Read the model definition and answer for the solid it produces. Units are mm, in the model's axes. Face numbers are marked on the shaded views. A direction names the side the tool comes from. Give positions to 0.01 mm unless a question says otherwise; leave off trailing zeros. Write each loop counter-clockwise with the first axis right and the second up, starting at its lowest first coordinate (ties: lowest second). Pieces come first, ordered by that corner, then holes. Notation, with made-up numbers: (19, 15) - (54, 15) arc R19 ccw to (54, 31) - close; hole circle Ø8 at (29.5, -4). An arc over 180 degrees is marked (long way). Answer as CSV lines item,"result".
```python
from build123d import *

# Parameters (mm, degrees)
SKETCH1_W            = 6
SKETCH1_H            = 6
BOSS_EXTRUDE1_DEPTH  = 3.61
SKETCH2_W            = 0.7
SKETCH2_H            = 0.3
BOSS_EXTRUDE2_DEPTH  = 2
SKETCH3_W            = 0.7
SKETCH3_H            = 1.35
BOSS_EXTRUDE3_DEPTH  = 1.15
SKETCH4_W            = 0.7
SKETCH4_H            = 0.3
BOSS_EXTRUDE4_DEPTH  = 2
SKETCH5_W            = 0.7
SKETCH5_H            = 1.35
BOSS_EXTRUDE5_DEPTH  = 1.15
SKETCH6_W            = 0.7
SKETCH6_H            = 0.3
BOSS_EXTRUDE6_DEPTH  = 2
SKETCH7_W            = 0.7
SKETCH7_H            = 1.35
BOSS_EXTRUDE7_DEPTH  = 1.15
SKETCH8_W            = 0.7
SKETCH8_H            = 0.3
BOSS_EXTRUDE8_DEPTH  = 2
SKETCH9_W            = 0.7
SKETCH9_H            = 1.35
BOSS_EXTRUDE9_DEPTH  = 1.15
CUT_EXTRUDE1_REACH   = 10.374
SKETCH10_W           = 1.15
SKETCH10_H           = 1.05
SKETCH11_W           = 1.15
SKETCH11_H           = 1.05
CUT_EXTRUDE2_DEPTH   = 8.923010791
CUT_EXTRUDE3_REACH   = 10.374
SKETCH12_W           = 1.15
SKETCH12_H           = 1.05
SKETCH13_W           = 1.15
SKETCH13_H           = 1.05
CUT_EXTRUDE4_DEPTH   = 8.923010791
SKETCH14_W           = 0.5
SKETCH14_H           = 0.4
SKETCH15_W           = 0.5
SKETCH15_H           = 0.4
SKETCH16_W           = 0.5
SKETCH16_H           = 0.4
SKETCH17_W           = 0.5
SKETCH17_H           = 0.4
FILLET1_R            = 0.25
FILLET2_R            = 0.55
SKETCH19_R           = 1.75
BOSS_EXTRUDE10_DEPTH = 1.4
FILLET4_R            = 0.1


with BuildPart() as part:
    # Sketch1 → Boss-Extrude1 (new body)
    with BuildSketch(Plane.XY):
        Rectangle(SKETCH1_W, SKETCH1_H)
    extrude(amount=-BOSS_EXTRUDE1_DEPTH)

    # Sketch2 → Boss-Extrude2 (add)
    with BuildSketch(Plane.XZ.offset(3)):
        with Locations((-2.25, -2.41)):
            Rectangle(SKETCH2_W, SKETCH2_H)
    extrude(amount=BOSS_EXTRUDE2_DEPTH)

    # Sketch3 → Boss-Extrude3 (add)
    with BuildSketch(Plane(origin=(0, 0, -2.56), x_dir=(-1, 0, 0), z_dir=(0, 0, -1))):
        with Locations((2.25, -4.325)):
            Rectangle(SKETCH3_W, SKETCH3_H)
    extrude(amount=BOSS_EXTRUDE3_DEPTH)

    # Sketch4 → Boss-Extrude4 (add)
    with BuildSketch(Plane.XZ.offset(3)):
        with Locations((2.25, -2.41)):
            Rectangle(SKETCH4_W, SKETCH4_H)
    extrude(amount=BOSS_EXTRUDE4_DEPTH)

    # Sketch5 → Boss-Extrude5 (add)
    with BuildSketch(Plane(origin=(0, 0, -2.56), x_dir=(-1, 0, 0), z_dir=(0, 0, -1))):
        with Locations((-2.25, -4.325)):
            Rectangle(SKETCH5_W, SKETCH5_H)
    extrude(amount=BOSS_EXTRUDE5_DEPTH)

    # Sketch6 → Boss-Extrude6 (add)
    with BuildSketch(Plane(origin=(0, 3, 0), x_dir=(-1, 0, 0), z_dir=(0, 1, 0))):
        with Locations((2.25, -2.41)):
            Rectangle(SKETCH6_W, SKETCH6_H)
    extrude(amount=BOSS_EXTRUDE6_DEPTH)

    # Sketch7 → Boss-Extrude7 (add)
    with BuildSketch(Plane(origin=(0, 0, -2.56), x_dir=(-1, 0, 0), z_dir=(0, 0, -1))):
        with Locations((2.25, 4.325)):
            Rectangle(SKETCH7_W, SKETCH7_H)
    extrude(amount=BOSS_EXTRUDE7_DEPTH)

    # Sketch8 → Boss-Extrude8 (add)
    with BuildSketch(Plane(origin=(0, 3, 0), x_dir=(-1, 0, 0), z_dir=(0, 1, 0))):
        with Locations((-2.25, -2.41)):
            Rectangle(SKETCH8_W, SKETCH8_H)
    extrude(amount=BOSS_EXTRUDE8_DEPTH)

    # Sketch9 → Boss-Extrude9 (add)
    with BuildSketch(Plane(origin=(0, 0, -2.56), x_dir=(-1, 0, 0), z_dir=(0, 0, -1))):
        with Locations((-2.25, 4.325)):
            Rectangle(SKETCH9_W, SKETCH9_H)
    extrude(amount=BOSS_EXTRUDE9_DEPTH)

    # Sketch10 → Cut-Extrude1 (cut, up to next)
    with BuildSketch(Plane.ZY.offset(2.6), mode=Mode.PRIVATE) as cut_extrude1_sk1:
        with Locations((-2.835, -4.475)):
            Rectangle(SKETCH10_W, SKETCH10_H)
    cut_extrude1_tool1 = extrude(cut_extrude1_sk1.sketch, amount=-CUT_EXTRUDE1_REACH, mode=Mode.PRIVATE) & part.part
    add(cut_extrude1_tool1.solids().sort_by_distance((-2.6, -4.475, -2.835))[0], mode=Mode.SUBTRACT)

    # Sketch11 → Cut-Extrude2 (cut, through all)
    with BuildSketch(Plane.ZY.offset(-1.9)):
        with Locations((-2.835, -4.475)):
            Rectangle(SKETCH11_W, SKETCH11_H)
    extrude(amount=-CUT_EXTRUDE2_DEPTH, mode=Mode.SUBTRACT)

    # Sketch12 → Cut-Extrude3 (cut, up to next)
    with BuildSketch(Plane.ZY.offset(2.6), mode=Mode.PRIVATE) as cut_extrude3_sk1:
        with Locations((-2.835, 4.475)):
            Rectangle(SKETCH12_W, SKETCH12_H)
    cut_extrude3_tool1 = extrude(cut_extrude3_sk1.sketch, amount=-CUT_EXTRUDE3_REACH, mode=Mode.PRIVATE) & part.part
    add(cut_extrude3_tool1.solids().sort_by_distance((-2.6, 4.475, -2.835))[0], mode=Mode.SUBTRACT)

    # Sketch13 → Cut-Extrude4 (cut, through all)
    with BuildSketch(Plane.ZY.offset(-1.9)):
        with Locations((-2.835, 4.475)):
            Rectangle(SKETCH13_W, SKETCH13_H)
    extrude(amount=-CUT_EXTRUDE4_DEPTH, mode=Mode.SUBTRACT)

    # Sketch14 → Revolve1 (revolve)
    with BuildSketch(Plane(origin=(0, -2.165, 0), x_dir=(-1, 0, 0), z_dir=(0, 1, 0))):
        with Locations((-2.415, 0.2)):
            Rectangle(SKETCH14_W, SKETCH14_H)
    revolve(axis=Axis((2.165, -2.165, 0), (0, 0, 1)))

    # Sketch15 → Revolve2 (revolve)
    with BuildSketch(Plane(origin=(0, -2.165, 0), x_dir=(-1, 0, 0), z_dir=(0, 1, 0))):
        with Locations((1.915, 0.2)):
            Rectangle(SKETCH15_W, SKETCH15_H)
    revolve(axis=Axis((-2.165, -2.165, 0), (0, 0, 1)))

    # Sketch16 → Revolve3 (revolve)
    with BuildSketch(Plane(origin=(0, 2.165, 0), x_dir=(-1, 0, 0), z_dir=(0, 1, 0))):
        with Locations((1.915, 0.2)):
            Rectangle(SKETCH16_W, SKETCH16_H)
    revolve(axis=Axis((-2.165, 2.165, 0), (0, 0, 1)))

    # Sketch17 → Revolve4 (revolve)
    with BuildSketch(Plane(origin=(0, 2.165, 0), x_dir=(-1, 0, 0), z_dir=(0, 1, 0))):
        with Locations((-2.415, 0.2)):
            Rectangle(SKETCH17_W, SKETCH17_H)
    revolve(axis=Axis((2.165, 2.165, 0), (0, 0, 1)))

    # Fillet1
    fillet1_edges = [part.edges().sort_by_distance(p)[0] for p in [
        (2.25, 3.65, -2.56),
        (-2.25, -3.95, -3.41),
        (2.25, -3.95, -3.41),
        (-2.25, 3.95, -3.41),
        (2.25, 3.95, -3.41),
        (-2.25, -3.65, -2.56),
        (2.25, -3.65, -2.56),
        (-3, -3, -1.805),
        (-3, 3, -1.805),
        (3, 3, -1.805),
        (3, -3, -1.805),
        (-2.25, 3.65, -2.56),
    ]]
    fillet(fillet1_edges, radius=FILLET1_R)

    # Fillet2
    fillet2_edges = [part.edges().sort_by_distance(p)[0] for p in [
        (2.25, 3.65, -3.71),
        (-2.25, -3.95, -2.26),
        (2.25, -3.95, -2.26),
        (-2.25, 3.95, -2.26),
        (2.25, 3.95, -2.26),
        (-2.25, -3.65, -3.71),
        (2.25, -3.65, -3.71),
        (-2.25, 3.65, -3.71),
    ]]
    fillet(fillet2_edges, radius=FILLET2_R)

    # Sketch19 → Boss-Extrude10 (add)
    with BuildSketch(Plane.XY):
        Circle(SKETCH19_R)
    extrude(amount=BOSS_EXTRUDE10_DEPTH)

    # Fillet4
    fillet4_edges = [part.edges().sort_by_distance(p)[0] for p in [
        (-1.75, 0, 1.4),
    ]]
    fillet(fillet4_edges, radius=FILLET4_R)


solid = part.part
```
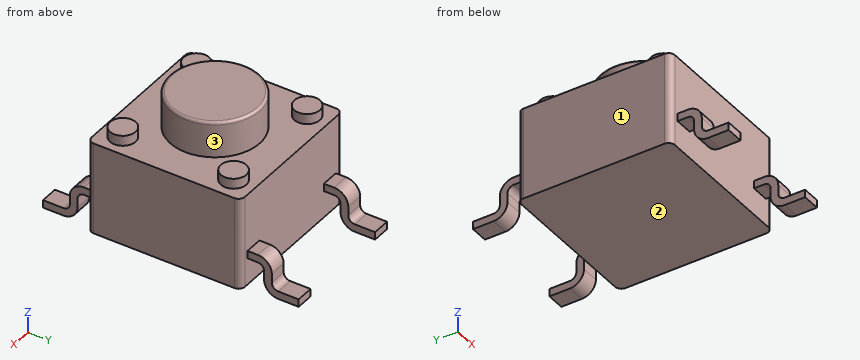
(1) A cutting plane is placed at A-A (x = 0). Write down the section's boundary in (y, z).
Worked out:
outline,"(-3, -3.61) - (3, -3.61) - (3, 0) - (1.75, 0) - (1.75, 1.3) arc R0.1 ccw to (1.65, 1.4) - (-1.65, 1.4) arc R0.1 ccw to (-1.75, 1.3) - (-1.75, 0) - (-3, 0) - close"
(2) Find the intervals of material crossed by L1, parallel to Y at x = -2.7, z = -0.65; L2, parallel to Z at x = -1.15, y = -0.5; L3, parallel to Z at x = 2.1, y = 3.25, in increasing order.
Worked out:
L1,"y = -3 to 3"
L2,"z = -3.61 to 1.4"
L3,"z = -2.56 to -2.26"
(3) Each of these flat-tipped pins is pushed along its axis until it touches: P1, Ø3, axis at x = 2.5, z = 0.5, coming from the +Y side; P2, Ø3, axis at x = -0.5, y = 1, coming from the -Z side; P3, Ø3, axis at x = -1, z = -1.5, coming from the +Y side. Where does it stop, or does it pass through?
Worked out:
P1,"stops at y = 3"
P2,"stops at z = -3.61"
P3,"stops at y = 3.94"
(4) A cutting plane is placed at B-B (z = -0.6). Write down the section's boundary in (x, y), and give its area (3 significant figures).
Worked out:
outline,"(-3, -2.75) arc R0.25 ccw to (-2.75, -3) - (2.75, -3) arc R0.25 ccw to (3, -2.75) - (3, 2.75) arc R0.25 ccw to (2.75, 3) - (-2.75, 3) arc R0.25 ccw to (-3, 2.75) - close"
area,"35.9 mm^2"
(5) A cutting plane is placed at D-D (z = -2.45). Write down the section's boundary in (x, y).
Worked out:
outline,"(-3, -2.75) arc R0.25 ccw to (-2.75, -3) - (-2.6, -3) - (-2.6, -3.82) - (-1.9, -3.82) - (-1.9, -3) - (1.9, -3) - (1.9, -3.82) - (2.6, -3.82) - (2.6, -3) - (2.75, -3) arc R0.25 ccw to (3, -2.75) - (3, 2.75) arc R0.25 ccw to (2.75, 3) - (2.6, 3) - (2.6, 3.82) - (1.9, 3.82) - (1.9, 3) - (-1.9, 3) - (-1.9, 3.82) - (-2.6, 3.82) - (-2.6, 3) - (-2.75, 3) arc R0.25 ccw to (-3, 2.75) - close"
(6) For the marked faces 1, 2 and 3, determine the directions among +Z, -Z, +X, -X, +Y, -Y from which every point of the face is accessible in a straight line to the end or side of a thin tool.
Worked out:
face 1,"+Z, -Z, -X, +Y, -Y"
face 2,"-Z, +X, -X"
face 3,"+Z"
